Verification items for the finished model (mm, model axes). Face numbers are marked on the shaded views. A direction names the side the tool comes from. Round coordinates to 2 decimals unless told otherwise and drop trailing zeros. Write each loop counter-clockwise with the first axis right and the second up, starting at its lowest first coordinate (ties: lowest second). Pieces come first, ordered by that corner, then holes. Notation, with made-up numbers: (-25, -40) - (31, -40) arc R24 cw to (31, -16) - close; hole circle Ø8 at (6.5, 87). An arc over 180 degrees is marked (long way). Write each question's results on one line, items separated by ' | '.
```python
from build123d import *

# Parameters (mm, degrees)
RESSALTO_EXTRUS_O1_DEPTH   = 25
CORTE_EXTRUS_O3_DEPTH      = 6
CORTE_EXTRUS_O3_DEPTH_BACK = 10
ESBO_O6_R                  = 1.65
CORTE_EXTRUS_O5_DEPTH      = 3
ESBO_O10_W                 = 0.5
ESBO_O10_H                 = 5
RESSALTO_EXTRUS_O3_DEPTH   = 6.7
RESSALTO_EXTRUS_O4_DEPTH   = 5
CORTE_EXTRUS_O6_START      = -1
CORTE_EXTRUS_O6_DEPTH      = 4
CHANFRO1_SIZE              = 6.4
ESBO_O13_R                 = 1.65
CORTE_EXTRUS_O7_DEPTH      = 13
CORTE_EXTRUS_O8_START      = -4
CORTE_EXTRUS_O8_DEPTH      = 10
CHANFRO2_SIZE              = 6.4


with BuildPart() as part:
    # Esboço1 → Ressalto-extrusão1 (new, symmetric)
    with BuildSketch(Plane.XY):
        with BuildLine():
            Line((0, 35), (0, -35))
            Line((0, -35), (13.5, -35))
            ThreePointArc((13.5, -35), (15.581665999, -34.780933834), (17.572127481, -34.133333333))
            Line((17.572127481, -34.133333333), (16.554095611, -31.85))
            ThreePointArc((16.554095611, -31.85), (6, -25), (16.554095611, -18.15))
            Line((16.554095611, -18.15), (17.572127481, -15.866666667))
            ThreePointArc((17.572127481, -15.866666667), (15.581665999, -15.219066166), (13.5, -15))
            Line((13.5, -15), (6, -15))
            Line((6, -15), (6, 15))
            Line((6, 15), (13.5, 15))
            ThreePointArc((13.5, 15), (15.581665999, 15.219066166), (17.572127481, 15.866666667))
            Line((17.572127481, 15.866666667), (16.554095611, 18.15))
            ThreePointArc((16.554095611, 18.15), (6, 25), (16.554095611, 31.85))
            Line((16.554095611, 31.85), (17.572127481, 34.133333333))
            ThreePointArc((17.572127481, 34.133333333), (15.581665999, 34.780933834), (13.5, 35))
            Line((13.5, 35), (0, 35))
        make_face()
    extrude(amount=RESSALTO_EXTRUS_O1_DEPTH, both=True)

    # Esboço6 → Corte-extrusão3 (cut, two sides: drawn at the far end of the back side and taken through both)
    with BuildSketch(Plane(origin=(6, 0, 0), x_dir=(0, 0, -1), z_dir=(1, 0, 0)).offset(-CORTE_EXTRUS_O3_DEPTH_BACK)):
        with Locations(Location((0, 11, 0), (0, 0, 180))):
            Circle(ESBO_O6_R)
        with Locations(Location((0, -11, 0), (0, 0, 180))):
            Circle(ESBO_O6_R)
        with Locations(Location((0, 0, 0), (0, 0, 180))):
            Circle(ESBO_O6_R)
    extrude(amount=CORTE_EXTRUS_O3_DEPTH + CORTE_EXTRUS_O3_DEPTH_BACK, mode=Mode.SUBTRACT)

    # Esboço9 → Corte-extrusão5 (cut)
    with BuildSketch(Plane.ZY):
        Polygon((3.175426481, 11), (1.58771324, 13.75), (-1.58771324, 13.75), (-3.175426481, 11), (-1.58771324, 8.25), (1.58771324, 8.25), align=None)
        Polygon((3.175426481, 0), (1.58771324, 2.75), (-1.58771324, 2.75), (-3.175426481, 0), (-1.58771324, -2.75), (1.58771324, -2.75), align=None)
        Polygon((3.175426481, -11), (1.58771324, -8.25), (-1.58771324, -8.25), (-3.175426481, -11), (-1.58771324, -13.75), (1.58771324, -13.75), align=None)
    extrude(amount=-CORTE_EXTRUS_O5_DEPTH, mode=Mode.SUBTRACT)

    # Esboço10 → Ressalto-extrusão3 (add)
    with BuildSketch(Plane.ZY):
        with Locations((-24.75, 25)):
            Rectangle(ESBO_O10_W, ESBO_O10_H)
        with Locations((24.75, 25)):
            Rectangle(ESBO_O10_W, ESBO_O10_H)
        with Locations((24.75, -25)):
            Rectangle(ESBO_O10_W, ESBO_O10_H)
        with Locations((-24.75, -25)):
            Rectangle(ESBO_O10_W, ESBO_O10_H)
    extrude(amount=-RESSALTO_EXTRUS_O3_DEPTH)

    # Esboço11 → Ressalto-extrusão4 (add)
    with BuildSketch(Plane.ZY):
        Polygon((-17.5, -7), (0, -14), (17.5, -7), (17.5, 26), (25, 26), (25, -16.924395537), (0, -26.924395537), (-25, -16.924395537), (-25, 26), (-17.5, 26), align=None)
    extrude(amount=RESSALTO_EXTRUS_O4_DEPTH)

    # Esboço12 → Corte-extrusão6 (cut)
    with BuildSketch(Plane.ZY.offset(5).offset(CORTE_EXTRUS_O6_START)):
        Polygon((-17.5, -7), (17.5, -7), (17.5, -14), (0, -21), (-17.5, -14), align=None)
    extrude(amount=-CORTE_EXTRUS_O6_DEPTH, mode=Mode.SUBTRACT)

    # Chanfro1
    # the kernel refuses this chamfer: 6.4 mm, written as the material it adds along each edge
    with BuildSketch(Plane(origin=(-4, -27.112634139, 15.281585348), x_dir=(0.9996219169112968, -0.025529280528386773, -0.01021171221135471), z_dir=(0, 0.3713906763541037, -0.9284766908852593))) as chanfro1_piece_1_section:
        Polygon((CHANFRO1_SIZE * 0.999621916911, -CHANFRO1_SIZE * 0.0274958766106), (-CHANFRO1_SIZE * 0.0274958766106, -CHANFRO1_SIZE * 0.999621916911), (0, 0), align=None)
    chanfro1_piece_1 = extrude(amount=51.765619071, mode=Mode.PRIVATE)
    chanfro1_piece_1 = split(chanfro1_piece_1, bisect_by=Plane(origin=(-1.981352532, -15.655988855, -17.5), z_dir=(0, 0, 1)), keep=Keep.TOP, mode=Mode.PRIVATE)
    chanfro1_piece_1 = split(chanfro1_piece_1, bisect_by=Plane(origin=(-1.981352532, -22.750248134, -4.375620334), z_dir=(0, 0.9284766908852595, -0.37139067635410344)), keep=Keep.TOP, mode=Mode.PRIVATE)
    add(chanfro1_piece_1)
    with BuildSketch(Plane(origin=(-4, -7.887365861, 32.781585348), x_dir=(0.9996219169112968, -0.02552928052838657, 0.010211712211354616), z_dir=(0, -0.37139067635410344, -0.9284766908852595))) as chanfro1_piece_2_section:
        Polygon((CHANFRO1_SIZE * 0.999621916911, -CHANFRO1_SIZE * 0.0274958766106), (-CHANFRO1_SIZE * 0.0274958766106, -CHANFRO1_SIZE * 0.999621916911), (0, 0), align=None)
    chanfro1_piece_2 = extrude(amount=51.765619071, mode=Mode.PRIVATE)
    chanfro1_piece_2 = split(chanfro1_piece_2, bisect_by=Plane(origin=(-1.981352532, -22.750248134, 4.375620334), z_dir=(0, 0.9284766908852595, 0.3713906763541038)), keep=Keep.TOP, mode=Mode.PRIVATE)
    chanfro1_piece_2 = split(chanfro1_piece_2, bisect_by=Plane(origin=(-1.981352532, -15.655988855, 17.5), z_dir=(0, 0, -1)), keep=Keep.TOP, mode=Mode.PRIVATE)
    add(chanfro1_piece_2)

    # Esboço13 → Corte-extrusão7 (cut)
    with BuildSketch(Plane.ZY):
        with Locations((0, 30.5)):
            Circle(ESBO_O13_R)
    extrude(amount=-CORTE_EXTRUS_O7_DEPTH, mode=Mode.SUBTRACT)

    # Esboço14 → Corte-extrusão8 (cut)
    with BuildSketch(Plane.ZY.offset(CORTE_EXTRUS_O8_START)):
        Polygon((3.175426481, 30.5), (1.58771324, 33.25), (-1.58771324, 33.25), (-3.175426481, 30.5), (-1.58771324, 27.75), (1.58771324, 27.75), align=None)
    extrude(amount=-CORTE_EXTRUS_O8_DEPTH, mode=Mode.SUBTRACT)

    # Chanfro2
    # the kernel refuses this chamfer: 6.4 mm, written as the material it adds along each edge
    with BuildSketch(Plane(origin=(0, -33.037029676, 15.281585348), x_dir=(-0.9996219169112968, 0.02552928052838658, 0.010211712211354642), z_dir=(0, 0.37139067635410405, -0.9284766908852592))) as chanfro2_piece_1_section:
        Polygon((CHANFRO2_SIZE * 0.999621916911, -CHANFRO2_SIZE * 0.0274958766106), (-CHANFRO2_SIZE * 0.0274958766106, -CHANFRO2_SIZE * 0.999621916911), (0, 0), align=None)
    chanfro2_piece_1 = extrude(amount=59.843366282, mode=Mode.PRIVATE)
    chanfro2_piece_1 = split(chanfro2_piece_1, bisect_by=Plane(origin=(-5, -23.598020322, -13.89468732), z_dir=(1, 0, 0)), keep=Keep.TOP, mode=Mode.PRIVATE)
    chanfro2_piece_1 = split(chanfro2_piece_1, bisect_by=Plane(origin=(-1.952897505, -23.598020322, -25), z_dir=(0, 0, 1)), keep=Keep.TOP, mode=Mode.PRIVATE)
    chanfro2_piece_1 = split(chanfro2_piece_1, bisect_by=Plane(origin=(-1.952897505, -31.256856652, -10.831152788), z_dir=(0, 0.9284766908852593, -0.3713906763541039)), keep=Keep.TOP, mode=Mode.PRIVATE)
    add(chanfro2_piece_1)
    with BuildSketch(Plane(origin=(0, -10.811761398, 40.281585348), x_dir=(-0.9996219169112968, 0.02552928052838644, -0.010211712211354581), z_dir=(0, -0.3713906763541039, -0.9284766908852593))) as chanfro2_piece_2_section:
        Polygon((CHANFRO2_SIZE * 0.999621916911, -CHANFRO2_SIZE * 0.0274958766106), (-CHANFRO2_SIZE * 0.0274958766106, -CHANFRO2_SIZE * 0.999621916911), (0, 0), align=None)
    chanfro2_piece_2 = extrude(amount=59.843366282, mode=Mode.PRIVATE)
    chanfro2_piece_2 = split(chanfro2_piece_2, bisect_by=Plane(origin=(-5, -23.598020322, 13.89468732), z_dir=(1, 0, 0)), keep=Keep.TOP, mode=Mode.PRIVATE)
    chanfro2_piece_2 = split(chanfro2_piece_2, bisect_by=Plane(origin=(-1.952897505, -23.598020322, 25), z_dir=(0, 0, -1)), keep=Keep.TOP, mode=Mode.PRIVATE)
    chanfro2_piece_2 = split(chanfro2_piece_2, bisect_by=Plane(origin=(-1.952897505, -31.256856652, 10.831152788), z_dir=(0, 0.9284766908852592, 0.37139067635410405)), keep=Keep.TOP, mode=Mode.PRIVATE)
    add(chanfro2_piece_2)
    with BuildSketch(Plane(origin=(0, -10.811761398, 40.281585348), x_dir=(-0.9996219169112968, 0.02552928052838644, -0.010211712211354581), z_dir=(0, -0.3713906763541039, -0.9284766908852593))) as chanfro2_piece_3a_section:
        Polygon((CHANFRO2_SIZE * 0.999621916911, -CHANFRO2_SIZE * 0.0274958766106), (-CHANFRO2_SIZE * 0.0274958766106, -CHANFRO2_SIZE * 0.999621916911), (0, 0), align=None)
    chanfro2_piece_3a = extrude(amount=59.843366282, mode=Mode.PRIVATE)
    chanfro2_piece_3a = split(chanfro2_piece_3a, bisect_by=Plane(origin=(-5, -31.260156378, -5.039042683), z_dir=(1, 0, 0)), keep=Keep.TOP, mode=Mode.PRIVATE)
    chanfro2_piece_3a = split(chanfro2_piece_3a, bisect_by=Plane(origin=(-1.927343951, -25.78483059, -2.848912368), z_dir=(0, -0.9284766908852592, -0.37139067635410405)), keep=Keep.TOP, mode=Mode.PRIVATE)
    chanfro2_piece_3a = split(chanfro2_piece_3a, bisect_by=Plane(origin=(-1.927343951, -35, -5.039042683), z_dir=(0, 1, 0)), keep=Keep.TOP, mode=Mode.PRIVATE)
    with BuildSketch(Plane(origin=(0, -33.037029676, 15.281585348), x_dir=(-0.9996219169112968, 0.02552928052838658, 0.010211712211354642), z_dir=(0, 0.37139067635410405, -0.9284766908852592))) as chanfro2_piece_3b_section:
        Polygon((CHANFRO2_SIZE * 0.999621916911, -CHANFRO2_SIZE * 0.0274958766106), (-CHANFRO2_SIZE * 0.0274958766106, -CHANFRO2_SIZE * 0.999621916911), (0, 0), align=None)
    chanfro2_piece_3b = extrude(amount=59.843366282, mode=Mode.PRIVATE)
    chanfro2_piece_3b = split(chanfro2_piece_3b, bisect_by=Plane(origin=(-5, -31.260156378, 5.039042683), z_dir=(1, 0, 0)), keep=Keep.TOP, mode=Mode.PRIVATE)
    chanfro2_piece_3b = split(chanfro2_piece_3b, bisect_by=Plane(origin=(-1.927343951, -25.78483059, 2.848912368), z_dir=(0, -0.9284766908852593, 0.3713906763541039)), keep=Keep.TOP, mode=Mode.PRIVATE)
    chanfro2_piece_3b = split(chanfro2_piece_3b, bisect_by=Plane(origin=(-1.927343951, -35, 5.039042683), z_dir=(0, 1, 0)), keep=Keep.TOP, mode=Mode.PRIVATE)
    chanfro2_piece_3 = chanfro2_piece_3a & chanfro2_piece_3b
    add(chanfro2_piece_3)


solid = part.part
```
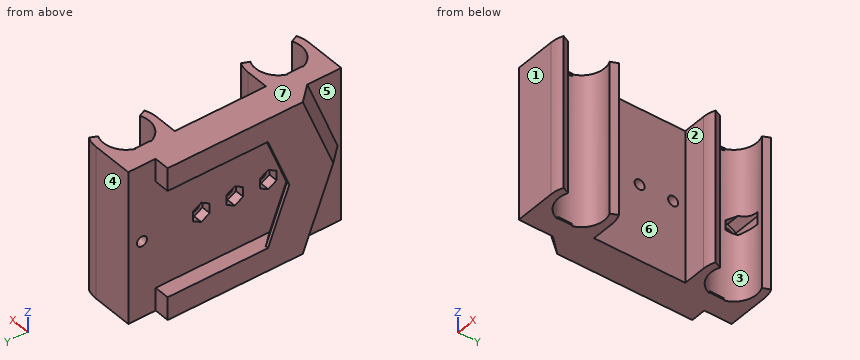
(1) Mould release check, pull along Y, two halves, no side actions. Record for the marked faces 1, 2, 3 and 4: released by +Y, released by -Y, zero draft, split by the parting line, or undercut.
Answer:
face 1: released by -Y | face 2: undercut | face 3: undercut | face 4: released by +Y
(2) Section check B-B (z = 20.5). Record the cut outline in (x, y).
Answer:
outline: (-5, -20.23) - (0, -25.62) - (0, -35) - (13.5, -35) arc R10 ccw to (17.57, -34.13) - (16.55, -31.85) arc R7.5 cw (long way) to (16.55, -18.15) - (17.57, -15.87) arc R10 ccw to (13.5, -15) - (6, -15) - (6, 15) - (13.5, 15) arc R10 ccw to (17.57, 15.87) - (16.55, 18.15) arc R7.5 cw (long way) to (16.55, 31.85) - (17.57, 34.13) arc R10 ccw to (13.5, 35) - (0, 35) - (0, 26) - (-5, 26) - close
(3) Set-up check for the marked faces 5, 6 and 7: record each of +Z, -Z, +X, -X, +Y, -Y from which the full face is reachable in a straight line by a thin tool's end or side.
Answer:
face 5: -X, -Y | face 6: +Z, -Z, +X | face 7: +Z, +X, -X, +Y, -Y
(4) Section check D-D (z = -11.5). Record the cut outline in (x, y), plus the area to 3 significant figures.
Answer:
outline: (-5, -23.83) - (0, -29.22) - (0, -35) - (13.5, -35) arc R10 ccw to (17.57, -34.13) - (16.55, -31.85) arc R7.5 cw (long way) to (16.55, -18.15) - (17.57, -15.87) arc R10 ccw to (13.5, -15) - (6, -15) - (6, 15) - (13.5, 15) arc R10 ccw to (17.57, 15.87) - (16.55, 18.15) arc R7.5 cw (long way) to (16.55, 31.85) - (17.57, 34.13) arc R10 ccw to (13.5, 35) - (0, 35) - (0, -13.82) - (-4, -9.51) - (-4, -9.4) - (-5, -9.4) - close | area: 657 mm2
(5) Thickness scan on L1, parallel to Y at x = 13.75, z = -14; L2, parallel to Y at x = 5.05, z = 0; L3, parallel to Y at x = 12.5, z = -20. Record the ranges inside material, lowest first.
Answer:
L1: -35 to -32.5, -17.5 to -15, 15 to 17.5, 32.5 to 35 | L2: -35 to -12.65, -9.35 to -1.65, 1.65 to 9.35, 12.65 to 27.75, 33.25 to 35 | L3: -35 to -32.43, -17.57 to -15, 15 to 17.57, 32.43 to 35
(6) Section check A-A (x = 10). Record the cut outline in (y, z).
Answer:
outline: (-35, -25) - (-31.63, -25) - (-31.63, 25) - (-35, 25) - close; (-18.37, -25) - (-15, -25) - (-15, 25) - (-18.37, 25) - close; (15, -25) - (18.37, -25) - (18.37, 25) - (15, 25) - close; (31.63, -25) - (35, -25) - (35, 25) - (31.63, 25) - (31.63, 2.52) - (33.25, 1.59) - (33.25, -1.59) - (31.63, -2.52) - close
(7) Section check C-C (y = -25). Record the cut outline in (x, z).
Answer:
outline: (-5, -8.58) - (0, -22.04) - (0, -25) - (6.7, -25) - (6.7, -24.5) - (6, -24.5) - (6, 24.5) - (6.7, 24.5) - (6.7, 25) - (0, 25) - (0, 22.04) - (-5, 8.58) - close
(8) Go/stop test with flat-tipped pins: pin 1 Ø1.6 at (y, z) = (-10, -1) entering from -X; pin 2 Ø6 at (y, z) = (-10.5, -10.5) entering from +X; pin 3 Ø5.5 at (y, z) = (30.5, 0) entering from -X. Record where each tip stops, or that it passes through.
Answer:
pin 1: x = 3 | pin 2: x = 6 | pin 3: x = 0
